Could you check a few things on this model? Use its own coordinates, in mm. A direction names the side the tool comes from. Give positions to 0.01 mm unless a question says otherwise; leave off trailing zeros. Write each loop counter-clockwise with the first axis right and the second up, starting at its lowest first coordinate (ties: lowest second). Pieces come first, ordered by that corner, then holes. Notation, with made-up numbers: M 42.25,48.25 L 99.25,48.25 A14 cw 99.25,66.25 Z; hole C 46.25,47.5 d6. An arc over 180 degrees is marked long. Use one line per item in the form item = value.
from build123d import *

# Parameters (mm, degrees)
BOSS_EXTRUDE1_DEPTH = 139.7
SKETCH2_R           = 12.7
CUT_EXTRUDE2_DEPTH  = 26.4


with BuildPart() as part:
    # Sketch1 → Boss-Extrude1 (new body)
    with BuildSketch(Plane(origin=(0, 0, 0), x_dir=(-1, 0, 0), z_dir=(0, 0, -1))):
        with BuildLine():
            Line((-12.7, 25.146), (-12.7, -25.146))
            ThreePointArc((-12.7, -25.146), (-12.625605122, -25.325605122), (-12.446, -25.4))
            Line((-12.446, -25.4), (12.446, -25.4))
            ThreePointArc((12.446, -25.4), (12.625605122, -25.325605122), (12.7, -25.146))
            Line((12.7, -25.146), (12.7, 25.146))
            ThreePointArc((12.7, 25.146), (12.625605122, 25.325605122), (12.446, 25.4))
            Line((12.446, 25.4), (-12.446, 25.4))
            ThreePointArc((-12.446, 25.4), (-12.625605122, 25.325605122), (-12.7, 25.146))
        make_face()
        with BuildLine():
            Line((-11.1125, -22.225), (-11.1125, 22.225))
            ThreePointArc((-11.1125, 22.225), (-10.647532015, 23.347532015), (-9.525, 23.8125))
            Line((-9.525, 23.8125), (9.525, 23.8125))
            ThreePointArc((9.525, 23.8125), (10.647532015, 23.347532015), (11.1125, 22.225))
            Line((11.1125, 22.225), (11.1125, -22.225))
            ThreePointArc((11.1125, -22.225), (10.647532015, -23.347532015), (9.525, -23.8125))
            Line((9.525, -23.8125), (-9.525, -23.8125))
            ThreePointArc((-9.525, -23.8125), (-10.647532015, -23.347532015), (-11.1125, -22.225))
        make_face(mode=Mode.SUBTRACT)
    extrude(amount=-BOSS_EXTRUDE1_DEPTH)

    # Sketch2 → Cut-Extrude2 (cut, through all)
    with BuildSketch(Plane(origin=(12.7, 0, 0), x_dir=(0, 0, -1), z_dir=(1, 0, 0))):
        with Locations((-115.282472, 0)):
            Circle(SKETCH2_R)
        with Locations((-24.417528, 0)):
            Circle(SKETCH2_R)
    extrude(amount=-CUT_EXTRUDE2_DEPTH, mode=Mode.SUBTRACT)


solid = part.part
1) For faces 1 (the flat face through (11.112, 0, 69)), 2 (the cylindrical face through (11.92, -7.73, 125.36)), which set-ups out of +Z, -Z, +X, -X, +Y, -Y let a thin tool reach every point of the face, with its end or its side?
Checked values:
face_1 = +Z, -Z
face_2 = +X, -X
2) I want a section at D-D, the plane y = 0. Please give me the cut outline in (x, z), plus the area to 3 significant figures.
Checked values:
outline = M -12.7,0 L -11.11,0 L -11.11,11.72 L -12.7,11.72 Z; M -12.7,37.12 L -11.11,37.12 L -11.11,102.58 L -12.7,102.58 Z; M -12.7,127.98 L -11.11,127.98 L -11.11,139.7 L -12.7,139.7 Z; M 11.11,0 L 12.7,0 L 12.7,11.72 L 11.11,11.72 Z; M 11.11,37.12 L 12.7,37.12 L 12.7,102.58 L 11.11,102.58 Z; M 11.11,127.98 L 12.7,127.98 L 12.7,139.7 L 11.11,139.7 Z
area = 282 mm2
3) I want a section at A-A, the plane x = -4.75. Please give me the cut outline in (y, z).
Checked values:
outline = M -25.4,0 L -23.81,0 L -23.81,139.7 L -25.4,139.7 Z; M 23.81,0 L 25.4,0 L 25.4,139.7 L 23.81,139.7 Z
4) Thinking about a two-plate mould opening in Z: for faces 3 (the flat face through (11.3, 2, 0)), 4 (the cylindrical face through (-11.9, -7.73, 125.36)), 5 (the flat face through (0, 25.4, 69)), which applies, released by +Z, released by -Z, zero draft, split by the parting line, or undercut?
Checked values:
face_3 = released by -Z
face_4 = undercut
face_5 = zero draft
5) If I drill on L1, parallel to X at y = 15, z = 54.5; L2, parallel to Y at x = 2.5, z = 110.5; L3, parallel to Y at x = -10, z = 121, over which ranges is the centre line in solid material (lowest first)?
Checked values:
L1 = -12.7 to -11.11, 11.11 to 12.7
L2 = -25.4 to -23.81, 23.81 to 25.4
L3 = -25.4 to -23.74, 23.74 to 25.4
6) I want a section at B-B, the plane y = 16. Please give me the cut outline in (x, z).
Checked values:
outline = M -12.7,0 L -11.11,0 L -11.11,139.7 L -12.7,139.7 Z; M 11.11,0 L 12.7,0 L 12.7,139.7 L 11.11,139.7 Z
